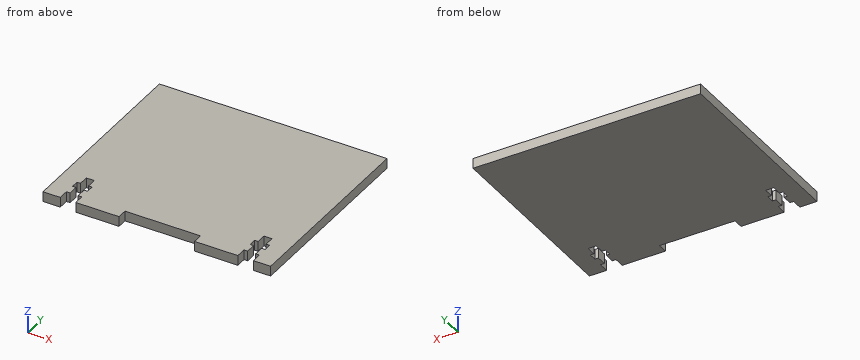
```python
from build123d import *

# Parameters (mm, degrees)
SKETCH1_W           = 91
SKETCH1_H           = 78.23
BOSS_EXTRUDE1_DEPTH = 4
CUT_EXTRUDE2_DEPTH  = 61.135124719
SKETCH3_W           = 30.2
SKETCH3_H           = 4
CUT_EXTRUDE3_DEPTH  = 4


with BuildPart() as part:
    # Sketch1 → Boss-Extrude1 (new body)
    with BuildSketch(Plane.XY):
        Rectangle(SKETCH1_W, SKETCH1_H)
    extrude(amount=BOSS_EXTRUDE1_DEPTH)

    # Sketch2 → Cut-Extrude2 (cut, through all)
    with BuildSketch(Plane.XY.offset(4)):
        Polygon((38.6, -39.115), (38.6, -35.015), (37.1, -35.015), (37.1, -31.015), (38.5, -31.015), (38.5, -28.015), (37.1, -28.015), (37.1, -24.115), (33.9, -24.115), (33.9, -28.015), (32.5, -28.015), (32.5, -31.015), (33.9, -31.015), (33.9, -35.015), (32.4, -35.015), (32.4, -39.115), align=None)
        Polygon((-32.4, -39.115), (-38.6, -39.115), (-38.6, -35.015), (-37.1, -35.015), (-37.1, -31.015), (-38.5, -31.015), (-38.5, -28.015), (-37.1, -28.015), (-37.1, -24.115), (-33.9, -24.115), (-33.9, -28.015), (-32.5, -28.015), (-32.5, -31.015), (-33.9, -31.015), (-33.9, -35.015), (-32.4, -35.015), align=None)
    extrude(amount=-CUT_EXTRUDE2_DEPTH, mode=Mode.SUBTRACT)

    # Sketch3 → Cut-Extrude3 (cut)
    with BuildSketch(Plane.XY.offset(4)):
        with Locations((0, -37.115)):
            Rectangle(SKETCH3_W, SKETCH3_H)
    extrude(amount=-CUT_EXTRUDE3_DEPTH, mode=Mode.SUBTRACT)


solid = part.part
```
Build history of the part. All positions in model axes, mm. Round coordinates to 2 decimals unless told otherwise and drop trailing zeros. Loops run counter-clockwise (first coordinate to the right, second up) from the corner with the lowest first, then second, coordinate; pieces in that order, holes last.
Item 1: Saw through at B-B (x = -1). List the corners of the cut face in (y, z) (3 decimals).
Item 2: Saw through at A-A (y = -34). List the corners of the cut face in (x, z).
Item 3: Pin check, flat tips, straight feed: P1, Ø1.5, axis at x = -37.5, z = 3, coming from the -Y side (3 decimals); P2, Ø1.6, axis at x = 35.5, z = 2, coming from the -Y side (3 decimals); P3, Ø1, axis at x = -3, z = 1, coming from the -Y side (3 decimals). Stop position of each tip, or through.
Item 4: Drill centre lines: line 1 along X through (y, z) = (-31.5, 0.8); line 2 along Y through (x, z) = (1, 3.3) (3 decimals); line 3 along Y through (x, z) = (35.5, 1.45) (3 decimals). Where is each one in solid material? Low to high.
Worked answers:
1. outline: (-35.115, 0) - (39.115, 0) - (39.115, 4) - (-35.115, 4) - close
2. outline: (-45.5, 0) - (-37.1, 0) - (-37.1, 4) - (-45.5, 4) - close; (-33.9, 0) - (33.9, 0) - (33.9, 4) - (-33.9, 4) - close; (37.1, 0) - (45.5, 0) - (45.5, 4) - (37.1, 4) - close
3. P1: stops at y = -35.015
3. P2: stops at y = -24.115
3. P3: stops at y = -35.115
4. line 1: x = -45.5 to -37.1, -33.9 to 33.9, 37.1 to 45.5
4. line 2: y = -35.115 to 39.115
4. line 3: y = -24.115 to 39.115
